from build123d import *

# Parameters (mm, degrees)
F0_W     = 168
F0_H     = 52
F1_DEPTH = 2
F2_W     = 168
F2_H     = 2
F3_DEPTH = 2
F5_DEPTH = 25
F6_W     = 2.6
F6_H     = 8.5
F7_DEPTH = 25


with BuildPart() as f1:
    # F0 (on Top) → F1 (new body)
    with BuildSketch(Plane.XY):
        Rectangle(F0_W, F0_H)
    extrude(amount=F1_DEPTH)

    # F2 (on face) → F3 (join)
    with BuildSketch(Plane.XY.offset(2)):
        with Locations((0, -27)):
            Rectangle(F2_W, F2_H)
        with Locations((0, -25)):
            Rectangle(F2_W, F2_H)
        with Locations((0, 25)):
            Rectangle(F2_W, F2_H)
        with Locations((0, 27)):
            Rectangle(F2_W, F2_H)
    extrude(amount=F3_DEPTH)

    # F4 (on face) → F5 (cut)
    with BuildSketch(Plane.XY.offset(2)):
        with BuildLine():
            ThreePointArc((78.5, -2), (78.369306, -1.387628), (78, -0.881966))
            ThreePointArc((78, -0.881966), (77, -0.5), (76, -0.881966))
            ThreePointArc((76, -0.881966), (76.387628, -3.369306), (78.5, -2))
        make_face()
        with BuildLine():
            Line((78, -0.881966), (78, 0.881966))
            ThreePointArc((78, 0.881966), (77, 0.5), (76, 0.881966))
            Line((76, 0.881966), (76, -0.881966))
            ThreePointArc((76, -0.881966), (77, -0.5), (78, -0.881966))
        make_face()
        with BuildLine():
            ThreePointArc((76, 0.881966), (77, 0.5), (78, 0.881966))
            ThreePointArc((78, 0.881966), (78.369306, 1.387628), (78.5, 2))
            ThreePointArc((78.5, 2), (76.387628, 3.369306), (76, 0.881966))
        make_face()
        with BuildLine():
            ThreePointArc((-78, -0.881966), (-77.612372, -3.369306), (-75.5, -2))
            ThreePointArc((-75.5, -2), (-75.630694, -1.387628), (-76, -0.881966))
            ThreePointArc((-76, -0.881966), (-77, -0.5), (-78, -0.881966))
        make_face()
        with BuildLine():
            ThreePointArc((-78, -0.881966), (-77, -0.5), (-76, -0.881966))
            Line((-76, -0.881966), (-76, 0.881966))
            ThreePointArc((-76, 0.881966), (-77, 0.5), (-78, 0.881966))
            Line((-78, 0.881966), (-78, -0.881966))
        make_face()
        with BuildLine():
            ThreePointArc((-78, 0.881966), (-77, 0.5), (-76, 0.881966))
            ThreePointArc((-76, 0.881966), (-75.630694, 1.387628), (-75.5, 2))
            ThreePointArc((-75.5, 2), (-77.612372, 3.369306), (-78, 0.881966))
        make_face()
    extrude(amount=-F5_DEPTH, mode=Mode.SUBTRACT)

    # F6 (on face) → F7 (cut)
    with BuildSketch(Plane.XY.offset(2)):
        with Locations((-82.7, 15.75)):
            Rectangle(F6_W, F6_H)
    extrude(amount=-F7_DEPTH, mode=Mode.SUBTRACT)


solid = f1.part
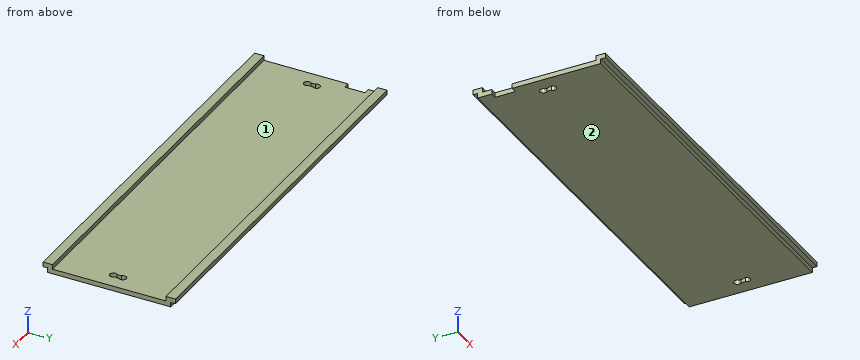
Could you check a few things on this model? Use its own coordinates, in mm. Face numbers are marked on the shaded views. Round coordinates to 2 decimals unless told otherwise and drop trailing zeros. Order: outer loops, then holes, each group sorted by start corner. A loop starts at its lowest first (then second) coordinate and runs counter-clockwise, first axis right, second up.
Q1. Imagine slicing it at A-A, the plane z = 1.4. List the corners of the cut face in (x, y) for me, then the cut area to 3 significant figures.
Geometry says:
outline: (-84, -26) - (84, -26) - (84, 26) - (-84, 26) - (-84, 20) - (-81.4, 20) - (-81.4, 11.5) - (-84, 11.5) - close; hole (-78, -0.88) arc R1.5 ccw (long way) to (-75.5, -2) arc R1.5 ccw to (-76, -0.88) - (-76, 0.88) arc R1.5 ccw to (-75.5, 2) arc R1.5 ccw (long way) to (-78, 0.88) - close; hole (76, -0.88) arc R1.5 ccw (long way) to (78.5, -2) arc R1.5 ccw to (78, -0.88) - (78, 0.88) arc R1.5 ccw to (78.5, 2) arc R1.5 ccw (long way) to (76, 0.88) - close
area: 8,680 mm2
Q2. Imagine slicing it at B-B, the plane x = -33.5. List the corners of the cut face in (y, z) for me.
Geometry says:
outline: (-28, 2) - (-26, 2) - (-26, 0) - (26, 0) - (26, 2) - (28, 2) - (28, 4) - (24, 4) - (24, 2) - (-24, 2) - (-24, 4) - (-28, 4) - close
Q3. I'm going to push flat-ended pins straight in: P1, Ø12, axis at x = 26.5, y = 1.5, coming from the +Z side; P2, Ø0.6, axis at x = -41.5, z = 1.5, coming from the +Y side; P3, Ø1.6, axis at y = 14, z = 1, coming from the -X side; P4, Ø10, axis at x = 10, y = 22, coming from the +Z side. Where does each tip first touch, or does it pass through?
Geometry says:
P1: stops at z = 2
P2: stops at y = 26
P3: stops at x = -81.4
P4: stops at z = 4
Q4. Please list where these lines run through material, in increasing order: probe 1 along X at (y, z) = (-2, 1.5); probe 2 along Y at (x, z) = (40, 3.35); probe 3 along Y at (x, z) = (77, 1.35).
Geometry says:
probe 1: x = -84 to -78.5, -75.5 to 75.5, 78.5 to 84
probe 2: y = -28 to -24, 24 to 28
probe 3: y = -26 to -3.5, 3.5 to 26
Q5. Imagine slicing it at C-C, the plane y = -20. List the corners of the cut face in (x, z) for me.
Geometry says:
outline: (-84, 0) - (84, 0) - (84, 2) - (-84, 2) - close
Q6. Thinking about a two-plate mould opening in Y: for the marked faces 1 and 2, which applies, released by +Y, released by -Y, zero draft, split by the parting line, or undercut?
Geometry says:
face 1: undercut
face 2: zero draft
